from build123d import *

# Parameters (mm, degrees)
FILLET1_R           = 0.2
SKETCH2_R           = 3.5
SKETCH2_R_2         = 3.15
BOSS_EXTRUDE1_DEPTH = 0.2


with BuildPart() as part:
    # Sketch1 → Revolve1 (revolve)
    with BuildSketch(Plane(origin=(0, 0, 0), x_dir=(0, 0, -1), z_dir=(1, 0, 0)), mode=Mode.PRIVATE) as revolve1_sk:
        Polygon((2.65, 1.25), (2.65, -1.25), (3.15, -1.25), (3.15, -1.05), (3.5, -1.05), (3.5, -1.25), (4, -1.25), (4, 1.25), (3.5, 1.25), (3.5, 1.05), (3.15, 1.05), (3.15, 1.25), align=None)
    revolve(revolve1_sk.sketch.rotate(Axis((0, 1.193675889, 0), (0, -1, 0)), 180), axis=Axis((0, 1.193675889, 0), (0, -1, 0)))

    # Fillet1
    fillet1_edges = [part.edges().sort_by_distance(p)[0] for p in [
        (0, 1.25, -4),
        (0, -1.25, -4),
        (0, -1.25, -2.65),
        (0, 1.25, -2.65),
    ]]
    fillet(fillet1_edges, radius=FILLET1_R)

    # Sketch2 → Boss-Extrude1 (add)
    with BuildSketch(Plane.XZ.offset(1.05)):
        with Locations(Location((0, 0, 0), (0, 0, 90))):
            Circle(SKETCH2_R)
        with Locations(Location((0, 0, 0), (0, 0, 90))):
            Circle(SKETCH2_R_2, mode=Mode.SUBTRACT)
    extrude(amount=BOSS_EXTRUDE1_DEPTH)


solid = part.part
Design review of the part built by this model. Coordinates are the model's own, in mm. Round coordinates to 2 decimals unless told otherwise and drop trailing zeros. Write each loop counter-clockwise with the first axis right and the second up, starting at its lowest first coordinate (ties: lowest second). Pieces come first, ordered by that corner, then holes.
Item 1: Consider section C-C on y = 0.7. Give the boundary of the cut face in (x, z).
Item 2: Wall thickness on L1, parallel to X at y = 1.1, z = 0; L2, parallel to X at y = -0.1, z = 2.25; L3, parallel to Z at x = 1.5, y = 1.15: over which ranges is each line inside the solid? List them lowest first.
Item 3: Draft analysis for pull direction X (two halves, no side actions). For faces 1 (the flat face through (-3, -1.25, 1)), 2 (the cylindrical face through (1.612, -0.015, -2.103)), 3 (the cylindrical face through (3.905, 0.015, -0.867)), state which applies: released by +X, released by -X, zero draft, split by the parting line, or undercut.
Item 4: Consider section A-A on x = 0. Give the boundary of the cut face in (y, z).
Item 5: Consider section B-B on z = 0. Give the boundary of the cut face in (x, y).
Item 6: For pin 1 Ø1.5 at (x, y) = (1, 0.5) entering from +Z; pin 2 Ø4 at (x, z) = (-1.5, -0.5) entering from +Y; pin 3 Ø1.5 at (y, z) = (-1, -2.5) entering from +X, all flat-tipped, find the tip position at first contact; note any pin that passes through.
Check values:
1. outline: circle Ø8 at (0, 0); hole circle Ø5.3 at (0, 0)
2. L1: x = -3.99 to -3.5, -3.15 to -2.66, 2.66 to 3.15, 3.5 to 3.99
2. L2: x = -3.31 to -1.4, 1.4 to 3.31
2. L3: z = -3.68 to -3.16, -2.77 to -2.22, 2.22 to 2.77, 3.16 to 3.68
3. face 1: zero draft
3. face 2: undercut
3. face 3: split by the parting line
4. outline: (-1.25, -3.8) arc R0.2 ccw to (-1.05, -4) - (1.05, -4) arc R0.2 ccw to (1.25, -3.8) - (1.25, -3.5) - (1.05, -3.5) - (1.05, -3.15) - (1.25, -3.15) - (1.25, -2.85) arc R0.2 ccw to (1.05, -2.65) - (-1.05, -2.65) arc R0.2 ccw to (-1.25, -2.85) - close; (-1.25, 2.85) arc R0.2 ccw to (-1.05, 2.65) - (1.05, 2.65) arc R0.2 ccw to (1.25, 2.85) - (1.25, 3.15) - (1.05, 3.15) - (1.05, 3.5) - (1.25, 3.5) - (1.25, 3.8) arc R0.2 ccw to (1.05, 4) - (-1.05, 4) arc R0.2 ccw to (-1.25, 3.8) - close
5. outline: (-4, -1.05) arc R0.2 ccw to (-3.8, -1.25) - (-2.85, -1.25) arc R0.2 ccw to (-2.65, -1.05) - (-2.65, 1.05) arc R0.2 ccw to (-2.85, 1.25) - (-3.15, 1.25) - (-3.15, 1.05) - (-3.5, 1.05) - (-3.5, 1.25) - (-3.8, 1.25) arc R0.2 ccw to (-4, 1.05) - close; (2.65, -1.05) arc R0.2 ccw to (2.85, -1.25) - (3.8, -1.25) arc R0.2 ccw to (4, -1.05) - (4, 1.05) arc R0.2 ccw to (3.8, 1.25) - (3.5, 1.25) - (3.5, 1.05) - (3.15, 1.05) - (3.15, 1.25) - (2.85, 1.25) arc R0.2 ccw to (2.65, 1.05) - close
6. pin 1: stops at z = 3.99
6. pin 2: stops at y = 1.25
6. pin 3: stops at x = 3.6
